```python
from build123d import *

# Parameters (mm, degrees)
F0_W     = 1000
F0_H     = 2000
F1_DEPTH = 25
F3_W     = 100
F3_H     = 725
F3_R     = 25
F4_DEPTH = 100


# Not quite as in the source:
# - a pattern or mirror of a feature is missing from the dataset's text; its kind, count and spacing are read off the source's solid


with BuildPart() as f1:
    # F0 (on Top) → F1 (new body)
    with BuildSketch(Plane.XY):
        with Locations((3.129221499, -3.3162072057)):
            Rectangle(F0_W, F0_H)
    extrude(amount=F1_DEPTH)

    # F3 (on offset) → F4 (join)
    with BuildSketch(Plane.YZ.offset(453.129221499)):
        with Locations((-903.3162072057, 387.5)):
            Rectangle(F3_W, F3_H)
        with Locations((-903.3162072057, 150)):
            Circle(F3_R, mode=Mode.SUBTRACT)
        with Locations((-903.3162072057, 350)):
            Circle(F3_R, mode=Mode.SUBTRACT)
        with Locations((-903.3162072057, 550)):
            Circle(F3_R, mode=Mode.SUBTRACT)
        with Locations((-103.3162072057, 387.5)):
            Rectangle(F3_W, F3_H)
        with Locations((-103.3162072057, 150)):
            Circle(F3_R, mode=Mode.SUBTRACT)
        with Locations((-103.3162072057, 350)):
            Circle(F3_R, mode=Mode.SUBTRACT)
        with Locations((-103.3162072057, 550)):
            Circle(F3_R, mode=Mode.SUBTRACT)
    f4 = extrude(amount=-F4_DEPTH)

    # F4_copies: F4 across plane
    add(f4.mirror(Plane(origin=(0, 0, 0), x_dir=(0, 0, -1), z_dir=(-1, 0, 0))))


solid = f1.part
```
The listing builds one solid part. Answer for the finished solid, in the listing's coordinates (mm). A direction names the side the tool comes from. Give positions to 0.01 mm unless a question says otherwise; leave off trailing zeros. Order: outer loops, then holes, each group sorted by start corner. A loop starts at its lowest first (then second) coordinate and runs counter-clockwise, first axis right, second up.
1) Consider line 1 along Z through (x, y) = (-393.5, -898.5); line 2 along Y through (x, z) = (384, 502.5); line 3 along X through (y, z) = (-898, 667). Determine where each line is inside the solid, lowest interval first.
Reported:
line 1: z = 0 to 125.47, 174.53 to 325.47, 374.53 to 525.47, 574.53 to 750
line 2: y = -953.32 to -853.32, -153.32 to -53.32
line 3: x = -453.13 to -353.13, 353.13 to 453.13
2) Find section C-C on y = -256. Write down the section's boundary in (x, z), then the cut area to 3 significant figures.
Reported:
outline: (-496.87, 0) - (503.13, 0) - (503.13, 25) - (-496.87, 25) - close
area: 25,000 mm2
3) For faces 4 (the face through (-404, -953.316, 382)), 5 (the face through (-353.129, -904, 393)), 6 (the face through (404, -153.316, 382)), determine the directions among +Z, -Z, +X, -X, +Y, -Y from which every point of the face is accessible in a straight line to the end or side of a thin tool.
Reported:
face 4: +Z, +X, -X, -Y
face 5: +Z, +Y, -Y
face 6: +Z, +X, -X
4) Find section D-D on x = -303. Write down the section's boundary in (y, z), then the cut area to 3 significant figures.
Reported:
outline: (-1003.32, 0) - (996.68, 0) - (996.68, 25) - (-1003.32, 25) - close
area: 50,000 mm2
5) Find section A-A on z = 271. Write down the section's boundary in (x, y).
Reported:
outline: (-453.13, -953.32) - (-353.13, -953.32) - (-353.13, -853.32) - (-453.13, -853.32) - close; (-453.13, -153.32) - (-353.13, -153.32) - (-353.13, -53.32) - (-453.13, -53.32) - close; (353.13, -953.32) - (453.13, -953.32) - (453.13, -853.32) - (353.13, -853.32) - close; (353.13, -153.32) - (453.13, -153.32) - (453.13, -53.32) - (353.13, -53.32) - close
6) Determine the mould class of faces 1 (the face through (404, -904, 750)), 2 (the face through (403.83, -879.47, 357.51)), 3 (the face through (-453.129, -904, 393)) for opening direction Z: pulls with the +Z half, pulls with the -Z half, needs draft (parallel to the pull), parting line crosses it, or undercut.
Reported:
face 1: pulls with the +Z half
face 2: undercut
face 3: needs draft
7) Find section B-B on z = 550. Give the number of separate pieces and of enclosed holes in the cut face, then the cut area to 3 significant figures.
Reported:
separate pieces: 8
enclosed holes: 0
area: 20,000 mm2
8) Given P1, Ø5, axis at x = 352.5, z = 585.5, coming from the -Y side, flat-ended and moving along its own axis, determine where the tip first touches the part or whether it passes through.
Reported:
P1: stops at y = -953.32
